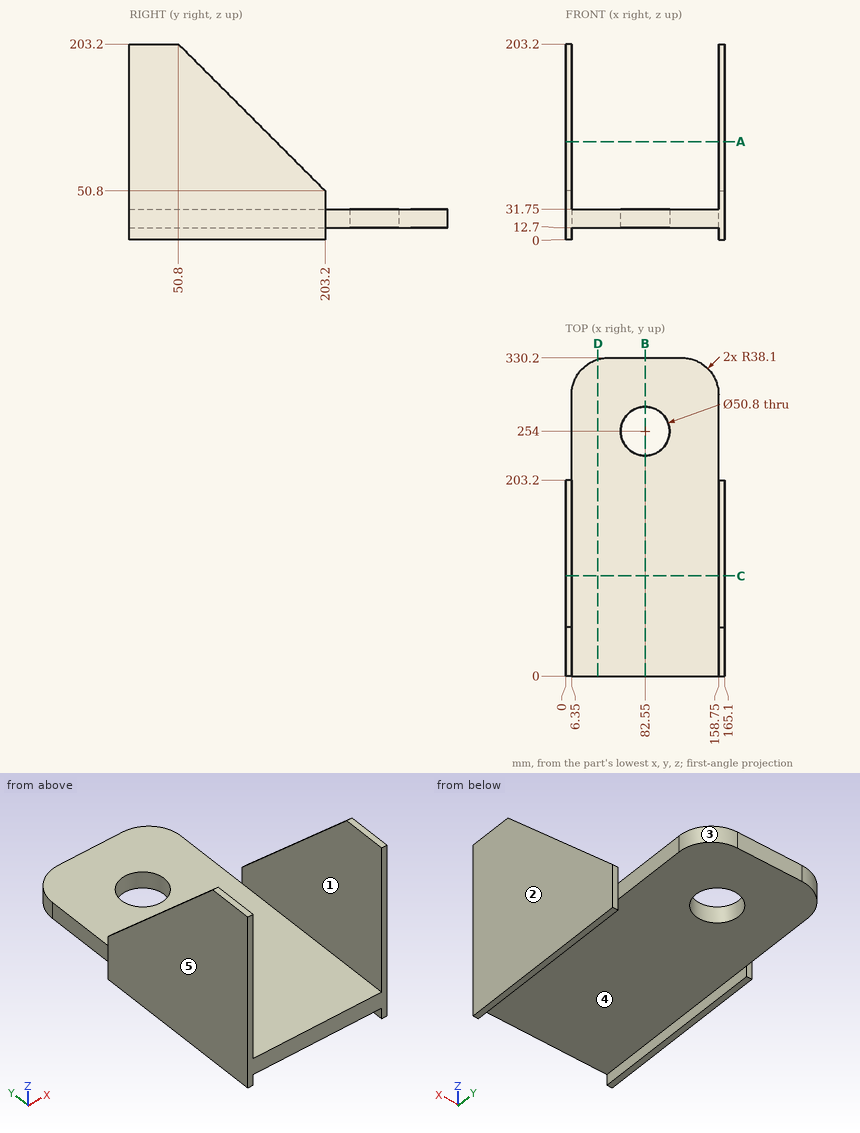
Verification items for this drawing (mm, ordinates from the low corner). A direction names the side the tool comes from. Coordinates: 2 decimals unless noted, no trailing zeros. Write each loop counter-clockwise with the first axis right and the second up, starting at its lowest first coordinate (ties: lowest second). Pieces come first, ordered by that corner, then holes. Notation, with made-up numbers: (49.5, -2.5) - (64.5, -2.5) arc R13 cw to (64.5, 21.5) - close; hole circle Ø7 at (64, 43). An arc over 180 degrees is marked (long way). One line per question, with ' | ' between items.
Item 1: Sectioned sample at B-B on x = 82.55. Record the boundary of the cut face in (y, z).
Determined:
outline: (0, 12.7) - (228.6, 12.7) - (228.6, 31.75) - (0, 31.75) - close; (279.4, 12.7) - (330.2, 12.7) - (330.2, 31.75) - (279.4, 31.75) - close
Item 2: Sectioned sample at C-C on y = 104. Record the boundary of the cut face in (x, z), plus the area to 3 significant figures.
Determined:
outline: (0, 0) - (6.35, 0) - (6.35, 12.7) - (158.75, 12.7) - (158.75, 0) - (165.1, 0) - (165.1, 150) - (158.75, 150) - (158.75, 31.75) - (6.35, 31.75) - (6.35, 150) - (0, 150) - close | area: 4,810 mm2
Item 3: Sectioned sample at D-D on x = 33.5. Record the boundary of the cut face in (y, z), plus the area to 3 significant figures.
Determined:
outline: (0, 12.7) - (328.59, 12.7) - (328.59, 31.75) - (0, 31.75) - close | area: 6,260 mm2
Item 4: Thickness scan on line 1 (Y direction, x = 82.55, z = 25.5); line 2 (X direction, y = 254, z = 17.5); line 3 (X direction, y = 90, z = 90). Record the ranges inside material, lowest first. Write a range as [from, to].
Determined:
line 1: y = [0, 228.6], [279.4, 330.2] | line 2: x = [6.35, 57.15], [107.95, 158.75] | line 3: x = [0, 6.35], [158.75, 165.1]
Item 5: Gauge pin test, flat ends, axial feed: P1, Ø3, axis at x = 2, z = 36, coming from the +Y side; P2, Ø10, axis at x = 75, y = 204.5, coming from the +Z side; P3, Ø5, axis at x = 72.5, y = 232, coming from the -Z side. Record the tip position at first contact, or that the pin passes through.
Determined:
P1: stops at y = 203.2 | P2: stops at z = 31.75 | P3: stops at z = 12.7
Item 6: Access from +Z, -Z, +X, -X, +Y, -Y to the whole of each face (thin tool, end or side, straight path). Record for the marked faces 1 and 2.
Determined:
face 1: +Z, +Y, -Y | face 2: +Z, -Z, +X, +Y, -Y
Item 7: Mould release check, pull along X, two halves, no side actions. Record for the marked faces 3, 4 and 5: pulls with the +X half, pulls with the -X half, needs draft (parallel to the pull), parting line crosses it, or undercut.
Determined:
face 3: pulls with the +X half | face 4: undercut | face 5: pulls with the -X half
Item 8: Sectioned sample at A-A on z = 102. Record the boundary of the cut face in (x, y).
Determined:
outline: (0, 0) - (6.35, 0) - (6.35, 152) - (0, 152) - close; (158.75, 0) - (165.1, 0) - (165.1, 152) - (158.75, 152) - close
